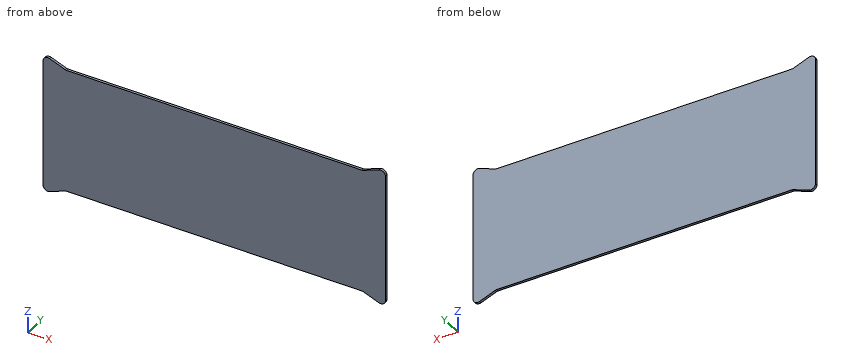
```python
from build123d import *

# Parameters (mm, degrees)
SKETCH1_W           = 412.75
SKETCH1_H           = 158.75
SKETCH1_R           = 6.191295591
BOSS_EXTRUDE1_DEPTH = 3.175
FILLET1_R           = 6.35


with BuildPart() as part:
    # Sketch1 → Boss-Extrude1 (new body)
    with BuildSketch(Plane(origin=(0, 0, 0), x_dir=(1, 0, 0), z_dir=(0, 1, 0))):
        with Locations((206.375, 79.375)):
            Rectangle(SKETCH1_W, SKETCH1_H)
        with Locations((418.528618537, 160.972545591)):
            Circle(SKETCH1_R)
        with BuildLine():
            Line((416.306072946, 166.751164128), (395.503046214, 158.75))
            Line((395.503046214, 158.75), (412.75, 158.75))
            ThreePointArc((412.75, 158.75), (412.870941125, 163.487068885), (416.306072946, 166.751164128))
        make_face()
        with BuildLine():
            Line((412.75, 158.75), (412.75, 0))
            ThreePointArc((412.75, 0), (419.658885237, 3.864706522), (424.719914128, -2.222545591))
            Line((424.719914128, -2.222545591), (424.719914128, 160.972545591))
            ThreePointArc((424.719914128, 160.972545591), (419.658885237, 154.885293478), (412.75, 158.75))
        make_face()
        with BuildLine():
            Line((412.75, 0), (395.503046214, 0))
            Line((395.503046214, 0), (416.306072946, -8.001164128))
            ThreePointArc((416.306072946, -8.001164128), (412.870941125, -4.737068885), (412.75, 0))
        make_face()
        with Locations((418.528618537, -2.222545591)):
            Circle(SKETCH1_R)
        with Locations((-5.778618537, 160.972545591)):
            Circle(SKETCH1_R)
        with BuildLine():
            ThreePointArc((0.412677054, 160.972545591), (0.308633576, 159.842278891), (0, 158.75))
            Line((0, 158.75), (17.246953786, 158.75))
            Line((17.246953786, 158.75), (-3.556072946, 166.751164128))
            ThreePointArc((-3.556072946, 166.751164128), (-0.675062041, 164.47766359), (0.412677054, 160.972545591))
        make_face()
        with BuildLine():
            ThreePointArc((-11.969914128, -2.222545591), (-6.908885237, 3.864706522), (0, 0))
            Line((0, 0), (0, 158.75))
            ThreePointArc((0, 158.75), (-6.908885237, 154.885293478), (-11.969914128, 160.972545591))
            Line((-11.969914128, 160.972545591), (-11.969914128, -2.222545591))
        make_face()
        with Locations((-5.778618537, -2.222545591)):
            Circle(SKETCH1_R)
        with BuildLine():
            Line((17.246953786, 0), (0, 0))
            ThreePointArc((0, 0), (0.308633576, -1.092278891), (0.412677054, -2.222545591))
            ThreePointArc((0.412677054, -2.222545591), (-0.675062041, -5.72766359), (-3.556072946, -8.001164128))
            Line((-3.556072946, -8.001164128), (17.246953786, 0))
        make_face()
    extrude(amount=BOSS_EXTRUDE1_DEPTH)

    # Fillet1
    fillet1_edges = [part.edges().sort_by_distance(p)[0] for p in [
        (17.246953786, 1.5875, -158.75),
        (395.503046214, 1.5875, -158.75),
        (395.503046214, 1.5875, 0),
        (17.246953786, 1.5875, 0),
    ]]
    fillet(fillet1_edges, radius=FILLET1_R)


solid = part.part
```
Geometry: final body of the model. Coordinates: model frame, mm. Coordinates: 2 decimals unless noted, no trailing zeros. Loops run counter-clockwise (first coordinate to the right, second up) from the corner with the lowest first, then second, coordinate; pieces in that order, holes last. Notation, with made-up numbers: (54.25, -26.5) -> (64.25, -26.5) arc R29 ccw to (64.25, 3.5) -> close; hole circle Ø4 at (8.25, 73.25). An arc over 180 degrees is marked (long way). Use a Markdown table: item, result. Add a question column.
(1) Section query A-A, the plane y = 2.65. Return loops of the section in (x, z), plus the area to 3 significant figures.
(2) Line query: line 1 along Z through (x, y) = (43, 1.7); line 2 along Z through (x, y) = (6.5, 3.05). Output: solid intervals per line, ascending.
(3) Section query B-B, the plane x = 271. Return loops of the section in (y, z) (3 decimals), plus the area to 3 significant figures.
(4) Pin query (flat end, axial travel): pin 1 Ø1.5 at (x, y) = (76, 0.5) entering from -Z; pin 2 Ø1 at (x, y) = (196.5, 2) entering from +Z. Return the tip coordinate at first contact, or that it passes through.
Answer:
| question | item | result |
|---|---|---|
| 1 | outline | (-11.97, -160.97) arc R6.19 ccw to (-3.56, -166.75) -> (16.15, -159.17) arc R6.35 cw to (18.43, -158.75) -> (394.32, -158.75) arc R6.35 cw to (396.6, -159.17) -> (416.31, -166.75) arc R6.19 ccw to (424.72, -160.97) -> (424.72, 2.22) arc R6.19 ccw to (416.31, 8) -> (396.6, 0.42) arc R6.35 cw to (394.32, 0) -> (18.43, 0) arc R6.35 cw to (16.15, 0.42) -> (-3.56, 8) arc R6.19 ccw to (-11.97, 2.22) -> close |
| 1 | area | 69,900 mm^2 |
| 2 | line 1 | z = -158.75 to 0 |
| 2 | line 2 | z = -162.88 to 4.13 |
| 3 | outline | (0, -158.75) -> (3.175, -158.75) -> (3.175, 0) -> (0, 0) -> close |
| 3 | area | 504 mm^2 |
| 4 | pin 1 | stops at z = -158.75 |
| 4 | pin 2 | stops at z = 0 |
